Work out the finished part from the listing and answer in its coordinate system (mm). Face numbers are marked on the shaded views. Round coordinates to 2 decimals unless told otherwise and drop trailing zeros. Loops run counter-clockwise (first coordinate to the right, second up) from the corner with the lowest first, then second, coordinate; pieces in that order, holes last. Notation, with made-up numbers: (-12, 15.5) -> (9, 15.5) arc R23 cw to (9, 42.5) -> close; hole circle Ø1 at (61.25, 67). An arc over 180 degrees is marked (long way). Write item = value, one per line. Start each with the question number.
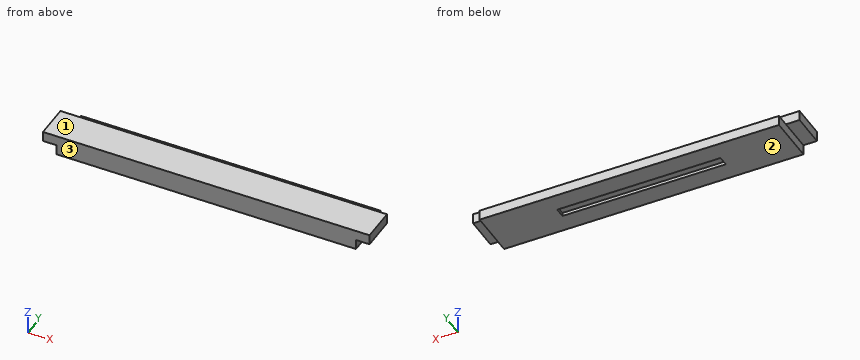
```python
from build123d import *

# Parameters (mm, degrees)
F0_W     = 558.8
F0_H     = 63.5
F0_W_2   = 304.8
F0_H_2   = 19.05
F0_W_3   = 25.4
F0_H_3   = 25.4
F1_DEPTH = 19.05
F2_DEPTH = 38.1
F3_DEPTH = 19.05
F4_DEPTH = 38.1
F5_DEPTH = 6.35


with BuildPart() as f1:
    # F0 (on Top) → F1 (new body)
    with BuildSketch(Plane.XY):
        with Locations((-15.767200847, -75.8242455751)):
            Rectangle(F0_W, F0_H)
        with Locations((-15.767200847, -63.1242455751)):
            Rectangle(F0_W_2, F0_H_2, mode=Mode.SUBTRACT)
        with Locations((-307.867200847, -75.8242455751)):
            Rectangle(F0_W_3, F0_H)
        with Locations((-15.767200847, -31.3742455751)):
            Rectangle(F0_W, F0_H_3)
        with Locations((276.332799153, -75.8242455751)):
            Rectangle(F0_W_3, F0_H)
    extrude(amount=F1_DEPTH)

    # F0 (on Top) → F2 (join)
    with BuildSketch(Plane.XY):
        with Locations((-15.767200847, -75.8242455751)):
            Rectangle(F0_W, F0_H)
        with Locations((-15.767200847, -63.1242455751)):
            Rectangle(F0_W_2, F0_H_2, mode=Mode.SUBTRACT)
        with Locations((-307.867200847, -75.8242455751)):
            Rectangle(F0_W_3, F0_H)
        with Locations((276.332799153, -75.8242455751)):
            Rectangle(F0_W_3, F0_H)
    extrude(amount=F2_DEPTH)

    # F0 (on Top) → F3 (cut)
    with BuildSketch(Plane.XY):
        with Locations((-307.867200847, -75.8242455751)):
            Rectangle(F0_W_3, F0_H)
        with Locations((276.332799153, -75.8242455751)):
            Rectangle(F0_W_3, F0_H)
    extrude(amount=F3_DEPTH, mode=Mode.SUBTRACT)

    # F0 (on Top) → F4 (join)
    with BuildSketch(Plane.XY):
        with Locations((-15.767200847, -63.1242455751)):
            Rectangle(F0_W_2, F0_H_2)
    extrude(amount=F4_DEPTH)

    # F0 (on Top) → F5 (cut)
    with BuildSketch(Plane.XY):
        with Locations((-15.767200847, -63.1242455751)):
            Rectangle(F0_W_2, F0_H_2)
    extrude(amount=F5_DEPTH, mode=Mode.SUBTRACT)


solid = f1.part
```
Item 1: The mould has two halves that part along Z. Classify the marked faces 1, 2 and 3: pulls with the +Z half, pulls with the -Z half, needs draft (parallel to the pull), parting line crosses it, or undercut.
Item 2: Section D-D (x = 202.5) is taken. Determine the outline of the cut face in (y, z).
Item 3: Section A-A (y = -82.5) is taken. Determine the outline of the cut face in (x, z), then the cut area to 3 significant figures.
Item 4: Find the intervals of material crossed by line 1 along Y through (x, z) = (194, 27.5); line 2 along Z through (x, y) = (85, -39.5); line 3 along Y through (x, z) = (42, 5), in increasing order. Write a range as [from, to].
Item 5: Section B-B (x = 27.5) is taken. Determine the outline of the cut face in (y, z), then the cut area to 3 significant figures.
Item 6: Flat-ended cylindrical pins translate along their axes: pin 1 (5.5 mm diameter, centred on y = -78.5, z = 9.5, fed in from -X); pin 2 (7.5 mm diameter, centred on x = -304.5, y = -65.5, fed in from -Z); pin 3 (1 mm diameter, centred on x = -161, z = 29, fed in from +Y). Find the tip coordinate at first contact, or state that the pin passes through.
Item 7: Section C-C (z = 24) is taken. Determine the outline of the cut face in (x, y).
Worked answers:
q1.face_1 = pulls with the +Z half
q1.face_2 = pulls with the -Z half
q1.face_3 = needs draft
q2.outline = (-107.57, 0) -> (-18.67, 0) -> (-18.67, 19.05) -> (-44.07, 19.05) -> (-44.07, 38.1) -> (-107.57, 38.1) -> close
q3.outline = (-320.57, 19.05) -> (-295.17, 19.05) -> (-295.17, 0) -> (263.63, 0) -> (263.63, 19.05) -> (289.03, 19.05) -> (289.03, 38.1) -> (-320.57, 38.1) -> close
q3.area = 22,300 mm2
q4.line_1 = [-107.57, -44.07]
q4.line_2 = [0, 19.05]
q4.line_3 = [-107.57, -72.65], [-53.6, -18.67]
q5.outline = (-107.57, 0) -> (-72.65, 0) -> (-72.65, 6.35) -> (-53.6, 6.35) -> (-53.6, 0) -> (-18.67, 0) -> (-18.67, 19.05) -> (-44.07, 19.05) -> (-44.07, 38.1) -> (-107.57, 38.1) -> close
q5.area = 2,780 mm2
q6.pin_1 = -295.17
q6.pin_2 = 19.05
q6.pin_3 = -44.07
q7.outline = (-320.57, -107.57) -> (289.03, -107.57) -> (289.03, -44.07) -> (-320.57, -44.07) -> close
